Geometry: final body of the model. Coordinates: model frame, mm. Round coordinates to 2 decimals unless told otherwise and drop trailing zeros. Order: outer loops, then holes, each group sorted by start corner. A loop starts at its lowest first (then second) coordinate and runs counter-clockwise, first axis right, second up. Notation, with made-up numbers: M 8,-32 L 35,-32 A20 ccw 35,-19 Z; hole C 69,8 d3. An arc over 180 degrees is marked long. Put each result on its own line as item: value. Start each with the question number.
1) Material intervals for probe 1 along Z at (x, y) = (-9, -6.25); probe 2 along Z at (x, y) = (20, -5.75); probe 3 along Y at (x, z) = (2, -14.5), sorted ascending. Write a range as [from, to].
2) Section C-C, the plane z = -10. Return loops of the section in (x, y).
3) Section B-B, the plane y = -3.5. Return loops of the section in (x, z).
4) Section D-D, the plane x = 2. Return loops of the section in (y, z), then the cut area to 3 significant figures.
5) Draft query along Z for faces 1 (the flat face through (5, 0, 5)), 2 (the flat face through (5, -5, 21)), 3 (the cylindrical face through (16.8, -4.9, -11.9)). Return one class per face: pulls with the +Z half, pulls with the -Z half, needs draft (parallel to the pull), parting line crosses it, or undercut.
6) Section A-A, the plane x = -9. Return loops of the section in (y, z), then the cut area to 3 significant figures.
7) First-contact query: P1, Ø4.5, axis at x = 9, z = -10, coming from the +Y side; P2, Ø0.9, axis at y = 0.5, z = -0.5, coming from the +X side. Flat tips, straight axial feed; report the tip coordinate or a pass-through.
from build123d import *

# Parameters (mm, degrees)
F0_R     = 3.2
F2_DEPTH = 10
F1_R     = 2
F3_DEPTH = 10
F4_W     = 40
F4_H     = 9.5
F5_DEPTH = 0.8


with BuildPart() as f2:
    # F0 (on Front) → F2 (new body)
    with BuildSketch(Plane.XZ):
        Polygon((-20, -21), (20, -21), (30, -21), (30, 21), (20, 21), (-20, 21), align=None)
        with Locations((20, -12)):
            Circle(F0_R, mode=Mode.SUBTRACT)
        with Locations((20, 12)):
            Circle(F0_R, mode=Mode.SUBTRACT)
    extrude(amount=F2_DEPTH)

    # F1 (on Front) → F3 (cut, through all)
    with BuildSketch(Plane.XZ):
        with Locations((-9, 10)):
            Circle(F1_R)
        with Locations((-9, -10)):
            Circle(F1_R)
        with Locations((9, 10)):
            Circle(F1_R)
        with Locations((9, -10)):
            Circle(F1_R)
    extrude(amount=F3_DEPTH, mode=Mode.SUBTRACT)

    # F4 (on face) → F5 (join)
    with BuildSketch(Plane(origin=(0, 0, 0), x_dir=(-1, 0, 0), z_dir=(0, 1, 0))):
        Rectangle(F4_W, F4_H)
    extrude(amount=F5_DEPTH)


solid = f2.part
Result sheet:
1. probe 1: z = [-21, -12], [-8, 8], [12, 21]
1. probe 2: z = [-21, -15.2], [-8.8, 8.8], [15.2, 21]
1. probe 3: y = [-10, 0]
2. outline: M -20,-10 L -11,-10 L -11,0 L -20,0 Z; M -7,-10 L 7,-10 L 7,0 L -7,0 Z; M 11,-10 L 17.5,-10 L 17.5,0 L 11,0 Z; M 22.5,-10 L 30,-10 L 30,0 L 22.5,0 Z
3. outline: M -20,-21 L 30,-21 L 30,21 L -20,21 Z; hole C -9,-10 d4; hole C -9,10 d4; hole C 9,-10 d4; hole C 9,10 d4; hole C 20,-12 d6.4; hole C 20,12 d6.4
4. outline: M -10,-21 L 0,-21 L 0,-4.75 L 0.8,-4.75 L 0.8,4.75 L 0,4.75 L 0,21 L -10,21 Z
4. area: 428 mm2
5. face 1: needs draft
5. face 2: pulls with the +Z half
5. face 3: undercut
6. outline: M -10,-21 L 0,-21 L 0,-12 L -10,-12 Z; M -10,-8 L 0,-8 L 0,-4.75 L 0.8,-4.75 L 0.8,4.75 L 0,4.75 L 0,8 L -10,8 Z; M -10,12 L 0,12 L 0,21 L -10,21 Z
6. area: 348 mm2
7. P1: stops at y = 0
7. P2: stops at x = 20
